Part model, mm, in its own coordinate system. Face numbers are marked on the shaded views. A direction names the side the tool comes from. Give positions to 0.01 mm unless a question says otherwise; leave off trailing zeros. Write each loop counter-clockwise with the first axis right and the second up, starting at its lowest first coordinate (ties: lowest second). Pieces come first, ordered by that corner, then holes. Notation, with made-up numbers: M 74.5,2 L 105.5,2 A26 ccw 105.5,17 Z; hole C 68.25,86 d11. An arc over 180 degrees is marked long. Write item = value, one per line. Start each with the question number.
from build123d import *
from OCP.BRepFilletAPI import BRepFilletAPI_MakeChamfer

# Parameters (mm, degrees)
BOSS_EXTRUDE1_DEPTH = 50
SKETCH5_W           = 63
SKETCH5_H           = 50
BOSS_EXTRUDE2_DEPTH = 1.6
CHAMFER6_SIZE       = 0.8
CHAMFER6_SIZE2      = 0.738449877
CHAMFER7_SIZE       = 0.8
CHAMFER7_SIZE2      = 0.880050294
CHAMFER7_SIZE2_2    = 0.59857957
FILLET1_R           = 7
CHAMFER10_SIZE      = 1.5
CUT_EXTRUDE5_REACH  = 79.922
CUT_EXTRUDE6_DEPTH  = 1.6


with BuildPart() as part:
    # Sketch1 → Boss-Extrude1 (new body)
    with BuildSketch(Plane.XY):
        Polygon((-34.595581798, 39), (-29.986555798, 39), (-32.97810591, 45.15618727), (-31.179250624, 46.030326652), (-27.76291945, 39), (-27.76291945, 37), (-32.76291945, 37), (-36, 0), (0, 0), (36, 0), (32.76291945, 37), (27.76291945, 37), (27.76291945, 39), (31.179250624, 46.030326652), (32.97810591, 45.15618727), (29.986555798, 39), (34.595581798, 39), (38.182617002, -2), (0, -2), (-38.182617002, -2), align=None)
    extrude(amount=BOSS_EXTRUDE1_DEPTH)

    # Sketch5 → Boss-Extrude2 (add)
    with BuildSketch(Plane.XZ.offset(2)):
        with Locations((0, 25)):
            Rectangle(SKETCH5_W, SKETCH5_H)
    extrude(amount=BOSS_EXTRUDE2_DEPTH)

    # Chamfer6: one chamfer whose edges measure the first distance from different faces: ONE call of the kernel's chamfer builder (chamfer() names one face for all edges)
    chamfer6_edges_1 = [part.edges().sort_by_distance(p)[0] for p in [
        (-36, 0, 25),
    ]]
    chamfer6_side_1 = [part.faces().sort_by_distance(p)[0] for p in [
        (0, 0, 25),
    ]]
    chamfer6_edges_2 = [part.edges().sort_by_distance(p)[0] for p in [
        (36, 0, 25),
    ]]
    chamfer6_side_2 = [part.faces().sort_by_distance(p)[0] for p in [
        (34.381459725, 18.5, 25),
    ]]
    chamfer6_edges_3 = [part.edges().sort_by_distance(p)[0] for p in [
        (38.182617002, -2, 25),
    ]]
    chamfer6_side_3 = [part.faces().sort_by_distance(p)[0] for p in [
        (34.841308501, -2, 25),
    ]]
    chamfer6_edges_4 = [part.edges().sort_by_distance(p)[0] for p in [
        (-38.182617002, -2, 25),
    ]]
    chamfer6_side_4 = [part.faces().sort_by_distance(p)[0] for p in [
        (-36.3890994, 18.5, 25),
    ]]
    chamfer6 = BRepFilletAPI_MakeChamfer(part.part.solid().wrapped)
    for e in chamfer6_edges_1:
        chamfer6.Add(CHAMFER6_SIZE, CHAMFER6_SIZE2, e.wrapped, chamfer6_side_1[0].wrapped)  # the first distance lies on this face
    for e in chamfer6_edges_2:
        chamfer6.Add(CHAMFER6_SIZE, CHAMFER6_SIZE2, e.wrapped, chamfer6_side_2[0].wrapped)  # the first distance lies on this face
    for e in chamfer6_edges_3:
        chamfer6.Add(CHAMFER6_SIZE, CHAMFER6_SIZE2, e.wrapped, chamfer6_side_3[0].wrapped)  # the first distance lies on this face
    for e in chamfer6_edges_4:
        chamfer6.Add(CHAMFER6_SIZE, CHAMFER6_SIZE2, e.wrapped, chamfer6_side_4[0].wrapped)  # the first distance lies on this face
    add(Compound.cast(chamfer6.Shape()), mode=Mode.REPLACE)

    # Chamfer7: one chamfer whose edges measure the first distance from different faces: ONE call of the kernel's chamfer builder (chamfer() names one face for all edges)
    chamfer7_edges_1 = [part.edges().sort_by_distance(p)[0] for p in [
        (-32.76291945, 37, 25),
    ]]
    chamfer7_side_1 = [part.faces().sort_by_distance(p)[0] for p in [
        (-34.349279651, 18.867819926, 25),
    ]]
    chamfer7_edges_2 = [part.edges().sort_by_distance(p)[0] for p in [
        (32.76291945, 37, 25),
    ]]
    chamfer7_side_2 = [part.faces().sort_by_distance(p)[0] for p in [
        (30.26291945, 37, 25),
    ]]
    chamfer7_edges_3 = [part.edges().sort_by_distance(p)[0] for p in [
        (29.986555798, 39, 25),
    ]]
    chamfer7_side_3 = [part.faces().sort_by_distance(p)[0] for p in [
        (32.291068798, 39, 25),
    ]]
    chamfer7_edges_4 = [part.edges().sort_by_distance(p)[0] for p in [
        (34.595581798, 39, 25),
    ]]
    chamfer7_side_4 = [part.faces().sort_by_distance(p)[0] for p in [
        (36.356919326, 18.867819926, 25),
    ]]
    chamfer7_edges_5 = [part.edges().sort_by_distance(p)[0] for p in [
        (-34.595581798, 39, 25),
    ]]
    chamfer7_side_5 = [part.faces().sort_by_distance(p)[0] for p in [
        (-32.291068798, 39, 25),
    ]]
    chamfer7_edges_6 = [part.edges().sort_by_distance(p)[0] for p in [
        (-29.986555798, 39, 25),
    ]]
    chamfer7_side_6 = [part.faces().sort_by_distance(p)[0] for p in [
        (-31.482330854, 42.078093635, 25),
    ]]
    chamfer7 = BRepFilletAPI_MakeChamfer(part.part.solid().wrapped)
    for e in chamfer7_edges_1:
        chamfer7.Add(CHAMFER7_SIZE, CHAMFER7_SIZE2, e.wrapped, chamfer7_side_1[0].wrapped)  # the first distance lies on this face
    for e in chamfer7_edges_2:
        chamfer7.Add(CHAMFER7_SIZE, CHAMFER7_SIZE2, e.wrapped, chamfer7_side_2[0].wrapped)  # the first distance lies on this face
    for e in chamfer7_edges_3:
        chamfer7.Add(CHAMFER7_SIZE, CHAMFER7_SIZE2_2, e.wrapped, chamfer7_side_3[0].wrapped)  # the first distance lies on this face
    for e in chamfer7_edges_4:
        chamfer7.Add(CHAMFER7_SIZE, CHAMFER7_SIZE2, e.wrapped, chamfer7_side_4[0].wrapped)  # the first distance lies on this face
    for e in chamfer7_edges_5:
        chamfer7.Add(CHAMFER7_SIZE, CHAMFER7_SIZE2, e.wrapped, chamfer7_side_5[0].wrapped)  # the first distance lies on this face
    for e in chamfer7_edges_6:
        chamfer7.Add(CHAMFER7_SIZE, CHAMFER7_SIZE2_2, e.wrapped, chamfer7_side_6[0].wrapped)  # the first distance lies on this face
    add(Compound.cast(chamfer7.Shape()), mode=Mode.REPLACE)

    # Fillet1
    fillet1_edges = [part.edges().sort_by_distance(p)[0] for p in [
        (-31.5, -2.8, 0),
        (31.5, -2.8, 0),
        (31.5, -2.8, 50),
        (-31.5, -2.8, 50),
    ]]
    fillet(fillet1_edges, radius=FILLET1_R)

    # Chamfer10
    chamfer10_edges = [part.edges().sort_by_distance(p)[0] for p in [
        (-31.5, -3.6, 25),
        (0, -3.6, 50),
        (0, -3.6, 0),
        (31.5, -3.6, 25),
        (29.449747468, -3.6, 47.949747468),
        (29.449747468, -3.6, 2.050252532),
        (-29.449747468, -3.6, 2.050252532),
        (-29.449747468, -3.6, 47.949747468),
    ]]
    chamfer(chamfer10_edges, length=CHAMFER10_SIZE)

    # Sketch15 → Cut-Extrude5 (cut, up to next)
    with BuildSketch(Plane(origin=(0, 0, 0), x_dir=(1, 0, 0), z_dir=(0, 1, 0)), mode=Mode.PRIVATE) as cut_extrude5_sk1:
        with BuildLine():
            Line((21.475016583, -42.866268583), (20.428249938, -41.819501939))
            ThreePointArc((20.428249938, -41.819501939), (16.022847213, -33.655561292), (24.186787861, -38.060964016))
            Line((24.186787861, -38.060964016), (25.233554505, -39.107730661))
            ThreePointArc((25.233554505, -39.107730661), (26.877324102, -44.51003818), (21.475016583, -42.866268583))
        make_face()
    cut_extrude5_tool1 = extrude(cut_extrude5_sk1.sketch, amount=-CUT_EXTRUDE5_REACH, mode=Mode.PRIVATE) & part.part
    # Sketch15 → Cut-Extrude5 (cut, up to next)
    with BuildSketch(Plane(origin=(0, 0, 0), x_dir=(1, 0, 0), z_dir=(0, 1, 0)), mode=Mode.PRIVATE) as cut_extrude5_sk2:
        with BuildLine():
            Line((-25.185393692, -39.138763585), (-24.139916413, -38.090709162))
            ThreePointArc((-24.139916413, -38.090709162), (-15.98140501, -33.675259948), (-20.37675457, -41.844617469))
            Line((-20.37675457, -41.844617469), (-21.422231849, -42.892671893))
            ThreePointArc((-21.422231849, -42.892671893), (-26.822511792, -44.543090495), (-25.185393692, -39.138763585))
        make_face()
    cut_extrude5_tool2 = extrude(cut_extrude5_sk2.sketch, amount=-CUT_EXTRUDE5_REACH, mode=Mode.PRIVATE) & part.part
    # Sketch15 → Cut-Extrude5 (cut, up to next)
    with BuildSketch(Plane(origin=(0, 0, 0), x_dir=(1, 0, 0), z_dir=(0, 1, 0)), mode=Mode.PRIVATE) as cut_extrude5_sk3:
        with BuildLine():
            Line((25.233554505, -10.892269339), (24.186787861, -11.939035984))
            ThreePointArc((24.186787861, -11.939035984), (16.022847213, -16.344438708), (20.428249938, -8.180498061))
            Line((20.428249938, -8.180498061), (21.475016583, -7.133731417))
            ThreePointArc((21.475016583, -7.133731417), (26.877324102, -5.48996182), (25.233554505, -10.892269339))
        make_face()
    cut_extrude5_tool3 = extrude(cut_extrude5_sk3.sketch, amount=-CUT_EXTRUDE5_REACH, mode=Mode.PRIVATE) & part.part
    # Sketch15 → Cut-Extrude5 (cut, up to next)
    with BuildSketch(Plane(origin=(0, 0, 0), x_dir=(1, 0, 0), z_dir=(0, 1, 0)), mode=Mode.PRIVATE) as cut_extrude5_sk4:
        with BuildLine():
            Line((-21.422231849, -7.107328107), (-20.37675457, -8.155382531))
            ThreePointArc((-20.37675457, -8.155382531), (-15.98140501, -16.324740052), (-24.139916413, -11.909290838))
            Line((-24.139916413, -11.909290838), (-25.185393692, -10.861236415))
            ThreePointArc((-25.185393692, -10.861236415), (-26.822511792, -5.456909505), (-21.422231849, -7.107328107))
        make_face()
    cut_extrude5_tool4 = extrude(cut_extrude5_sk4.sketch, amount=-CUT_EXTRUDE5_REACH, mode=Mode.PRIVATE) & part.part
    add(cut_extrude5_tool1.solids().sort_by_distance((21.014912, 0, 38.647626))[0], mode=Mode.SUBTRACT)
    add(cut_extrude5_tool2.solids().sort_by_distance((-20.96732, 0, 38.673466))[0], mode=Mode.SUBTRACT)
    add(cut_extrude5_tool3.solids().sort_by_distance((21.014912, 0, 11.352374))[0], mode=Mode.SUBTRACT)
    add(cut_extrude5_tool4.solids().sort_by_distance((-20.96732, 0, 11.326534))[0], mode=Mode.SUBTRACT)

    # Sketch16 → Cut-Extrude6 (cut)
    with BuildSketch(Plane(origin=(0, 0, 0), x_dir=(1, 0, 0), z_dir=(0, 1, 0))):
        with BuildLine():
            Line((-15.951616609, -40.543181032), (-21.113676241, -45.71796535))
            ThreePointArc((-21.113676241, -45.71796535), (-28.002957525, -45.726446075), (-28.011438251, -38.837164791))
            Line((-28.011438251, -38.837164791), (-22.849378618, -33.662380473))
            ThreePointArc((-22.849378618, -33.662380473), (-15.960097334, -33.653899748), (-15.951616609, -40.543181032))
        make_face()
        with BuildLine():
            Line((-15.951616609, -9.456818968), (-21.113676241, -4.28203465))
            ThreePointArc((-21.113676241, -4.28203465), (-28.002957525, -4.273553925), (-28.011438251, -11.162835209))
            Line((-28.011438251, -11.162835209), (-22.849378618, -16.337619527))
            ThreePointArc((-22.849378618, -16.337619527), (-15.960097334, -16.346100252), (-15.951616609, -9.456818968))
        make_face()
        with BuildLine():
            Line((15.951616609, -40.543181032), (21.113676241, -45.71796535))
            ThreePointArc((21.113676241, -45.71796535), (28.002957525, -45.726446075), (28.011438251, -38.837164791))
            Line((28.011438251, -38.837164791), (22.849378618, -33.662380473))
            ThreePointArc((22.849378618, -33.662380473), (15.960097334, -33.653899748), (15.951616609, -40.543181032))
        make_face()
        with BuildLine():
            Line((15.951616609, -9.456818968), (21.113676241, -4.28203465))
            ThreePointArc((21.113676241, -4.28203465), (28.002957525, -4.273553925), (28.011438251, -11.162835209))
            Line((28.011438251, -11.162835209), (22.849378618, -16.337619527))
            ThreePointArc((22.849378618, -16.337619527), (15.960097334, -16.346100252), (15.951616609, -9.456818968))
        make_face()
    extrude(amount=-CUT_EXTRUDE6_DEPTH, mode=Mode.SUBTRACT)


solid = part.part
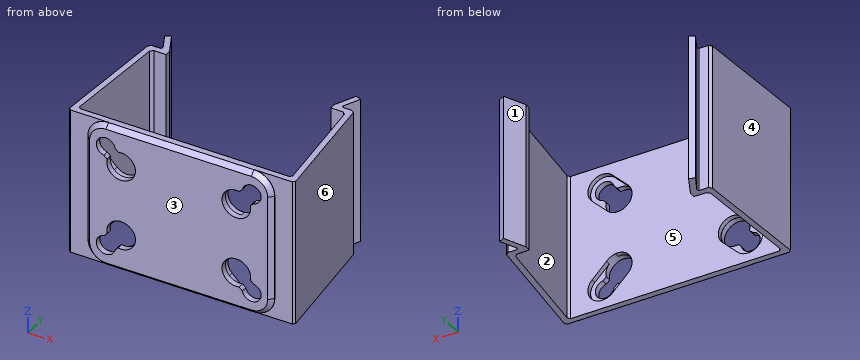
Q1. Slice it at D-D (z = 35.5). Give the number of separate pieces and of enclosed holes in the cut face, and give its area (3 significant figures).
Q2. Two-plate mould, pull along X, no slides. Class the marked faces 3, 4, 5 and 6: +X half, -X half, draft (parallel to the pull), parting line (faces both ways), or undercut.
Q3. Slice it at C-C (x = 1.5). Give the cut face in (y, z).
Q4. Probe line 1 along Y through (x, z) = (-17, 4.5); line 2 along Y through (x, z) = (19.5, 43.5); line 3 along X through (y, z) = (26.5, 46). List the from-to ranges inside material, lowest first.
Q5. Tool access for the marked faces 1 and 2: list every direction of +Z, -Z, +X, -X, +Y, -Y with a clear straight run to the whole face (end or side of a thin tool).
Q6. Drop flat-ended pins along their axis: P1, Ø16.5, axis at x = -19, z = 42, coming from the +Y side; P2, Ø12, axis at y = 9, z = 13.5, coming from the +X side; P3, Ø7.5, axis at x = 24.61, z = 42.25, coming from the -Y side; P4, Ø5, axis at y = 25.5, z = 15, coming from the -X side. Give the stop position or say it passes through.
Q7. Slice it at B-B (y = 14). Give the cut face in (x, z), and give its area (3 significant figures).
Working result:
q1.separate_pieces = 3
q1.enclosed_holes = 0
q1.area = 389 mm2
q2.face_3 = draft
q2.face_4 = -X half
q2.face_5 = undercut
q2.face_6 = +X half
q3.outline = M -3.6,1.5 L -2.1,0 L 0,0 L 0,50 L -2.1,50 L -3.6,48.5 Z
q4.line_1 = -3.6 to 0
q4.line_2 = -3.6 to -1.6
q4.line_3 = -35.69 to -33.68, 33.68 to 35.69
q5.face_1 = +Z, -Z, +Y
q5.face_2 = +Z, -Z
q6.P1 = 0
q6.P2 = 37.75
q6.P3 = -3.6
q6.P4 = -36
q7.outline = M -36.78,0 L -34.78,0 L -34.78,50 L -36.78,50 Z; M 34.78,0 L 36.78,0 L 36.78,50 L 34.78,50 Z
q7.area = 201 mm2
